```python
from build123d import *

# Parameters (mm, degrees)
SKETCH1_W                    = 139.7
SKETCH1_H                    = 457.2
SKETCH1_R                    = 50.8
SKETCH1_R_2                  = 5.08
BOSS_EXTRUDE1_DEPTH          = 9.652
SKETCH4_W                    = 10.452383168
SKETCH4_H                    = 6.858
SKETCH4_W_2                  = 8.864883168
SKETCH4_H_2                  = 6.35
CUT_EXTRUDE1_DEPTH           = 10.652
CHAMFER1_SIZE                = 15.24
CHAMFER1_SIZE2               = 30.48
CHAMFER2_SIZE                = 30.48
CHAMFER2_SIZE2               = 15.24
FILLET2_R                    = 15.24
SKETCH5_W                    = 76.2
SKETCH5_H                    = 9.652
BOSS_EXTRUDE2_DEPTH          = 4.318
F_3_0_3_DIAMETER_HOLE1_D     = 3
F_3_0_3_DIAMETER_HOLE1_DEPTH = 9.652


with BuildPart() as part:
    # Sketch1 → Boss-Extrude1 (new body)
    with BuildSketch(Plane(origin=(0, 0, 0), x_dir=(1, 0, 0), z_dir=(0, 1, 0))):
        with Locations((69.85, 228.6)):
            Rectangle(SKETCH1_W, SKETCH1_H)
        with Locations((63.5, 125.73)):
            Circle(SKETCH1_R, mode=Mode.SUBTRACT)
        with Locations((38.1, 38.1)):
            Circle(SKETCH1_R_2, mode=Mode.SUBTRACT)
        with Locations((38.1, 419.1)):
            Circle(SKETCH1_R_2, mode=Mode.SUBTRACT)
        with Locations((63.5, 331.47)):
            Circle(SKETCH1_R, mode=Mode.SUBTRACT)
        with Locations((38.1, 228.6)):
            Circle(SKETCH1_R_2, mode=Mode.SUBTRACT)
    extrude(amount=BOSS_EXTRUDE1_DEPTH)

    # Sketch4 → Cut-Extrude1 (cut, through all)
    with BuildSketch(Plane(origin=(0, 9.652, 0), x_dir=(1, 0, 0), z_dir=(0, 1, 0))):
        with Locations((5.226191584, 3.429)):
            Rectangle(SKETCH4_W, SKETCH4_H)
        with Locations((4.432441584, 454.025)):
            Rectangle(SKETCH4_W_2, SKETCH4_H_2)
    extrude(amount=-CUT_EXTRUDE1_DEPTH, mode=Mode.SUBTRACT)

    # Chamfer1
    chamfer1_edges = [part.edges().sort_by_distance(p)[0] for p in [
        (139.7, 4.826, -457.2),
    ]]
    chamfer1_side = [part.faces().sort_by_distance(p)[0] for p in [
        (139.7, 4.826, -228.6),
    ]]
    chamfer(chamfer1_edges, length=CHAMFER1_SIZE, length2=CHAMFER1_SIZE2, reference=chamfer1_side[0])

    # Chamfer2
    chamfer2_edges = [part.edges().sort_by_distance(p)[0] for p in [
        (139.7, 4.826, 0),
    ]]
    chamfer2_side = [part.faces().sort_by_distance(p)[0] for p in [
        (75.076191584, 4.826, 0),
    ]]
    chamfer(chamfer2_edges, length=CHAMFER2_SIZE, length2=CHAMFER2_SIZE2, reference=chamfer2_side[0])

    # Fillet2
    fillet2_edges = [part.edges().sort_by_distance(p)[0] for p in [
        (109.22, 4.826, -457.2),
        (109.22, 4.826, 0),
    ]]
    fillet(fillet2_edges, radius=FILLET2_R)

    # Sketch5 → Boss-Extrude2 (add)
    with BuildSketch(Plane(origin=(139.7, 0, 0), x_dir=(0, 0, -1), z_dir=(1, 0, 0))):
        with Locations((69.85, 4.826)):
            Rectangle(SKETCH5_W, SKETCH5_H)
        with Locations((228.6, 4.826)):
            Rectangle(SKETCH5_W, SKETCH5_H)
        with Locations((387.35, 4.826)):
            Rectangle(SKETCH5_W, SKETCH5_H)
    extrude(amount=BOSS_EXTRUDE2_DEPTH)

    # Ø3.0 (3) Diameter Hole1
    with Locations(Plane(origin=(0, 9.652, 0), x_dir=(1, 0, 0), z_dir=(0, 1, 0))):
        with Locations((101.092, 87.884), (25.4, 87.884), (25.4, 163.576), (101.092, 163.576)):
            f_3_0_3_diameter_hole1 = Hole(F_3_0_3_DIAMETER_HOLE1_D / 2, depth=F_3_0_3_DIAMETER_HOLE1_DEPTH)

    # Mirror1: Ø3.0 (3) Diameter Hole1 across plane
    add(f_3_0_3_diameter_hole1.mirror(Plane.XY.offset(-228.6)), mode=Mode.SUBTRACT)


solid = part.part
```
The listing builds one solid part. Answer for the finished solid, in the listing's coordinates (mm). A direction names the side the tool comes from. Coordinates: 2 decimals unless noted, no trailing zeros. Loops run counter-clockwise (first coordinate to the right, second up) from the corner with the lowest first, then second, coordinate; pieces in that order, holes last. Notation, with made-up numbers: (-36, -31) - (9, -31) arc R9 ccw to (9, -24) - close; hole circle Ø9 at (52, -31). An arc over 180 degrees is marked (long way). Use a Markdown table: item, result. Add a question column.
1) The part is cut by section A-A, the plane z = -228.6. Give the vertices of the cut face in (x, y).
2) Given pin 1 (2.5 mm diameter, centred on x = 101.092, z = -369.316, fed in from +Y); pin 2 (5 mm diameter, centred on y = 5, z = -23.5, fed in from +X); pin 3 (1.3 mm diameter, centred on x = 141, y = 3, fed in from -Z); pin 4 (5.5 mm diameter, centred on y = 6, z = -3.5, fed in from -X), each flat-ended and moving along its own axis, determine where each tip first touches the part or whether it passes through.
3) The part is cut by section D-D, the plane x = 38.1. Give the vertices of the cut face in (y, z).
4) The part is cut by section C-C, the plane z = -331.47. Give the vertices of the cut face in (x, y), and give its area (3 significant figures).
5) The part is cut by section B-B, the plane x = 63.5. Give the vertices of the cut face in (y, z), and give its area (3 significant figures).
6) The mould has two halves that part along Z. Classify faces 1 (the flat face through (126.26, 4.76, -8.52)), 2 (the flat face through (139.7, 5, -434)), 3 (the cylindrical face through (26, 5, -160)): released by +Z, released by -Z, zero draft, split by the parting line, or undercut.
7) For faces 4 (the flat face through (4, 5, -450.85)), 5 (the flat face through (139.7, 5, -307)), 6 (the flat face through (5, 5, -6.858)), 7 (the flat face through (139.7, 5, -23)), determine the directions among +Z, -Z, +X, -X, +Y, -Y from which every point of the face is accessible in a straight line to the end or side of a thin tool.
8) Find the intervals of material crossed by line 1 (Z direction, x = 63.5, y = 2); line 2 (X direction, y = 7.5, z = -331.47); line 3 (X direction, y = 3, z = -38.1), in increasing order.
Here are the results:
| question | item | result |
|---|---|---|
| 1 | outline | (0, 0) - (33.02, 0) - (33.02, 9.65) - (0, 9.65) - close; (43.18, 0) - (144.02, 0) - (144.02, 9.65) - (43.18, 9.65) - close |
| 2 | pin 1 | passes through |
| 2 | pin 2 | stops at x = 139.7 |
| 2 | pin 3 | stops at z = -425.45 |
| 2 | pin 4 | stops at x = 10.45 |
| 3 | outline | (0, -457.2) - (9.65, -457.2) - (9.65, -424.18) - (0, -424.18) - close; (0, -414.02) - (9.65, -414.02) - (9.65, -375.46) - (0, -375.46) - close; (0, -287.48) - (9.65, -287.48) - (9.65, -233.68) - (0, -233.68) - close; (0, -223.52) - (9.65, -223.52) - (9.65, -169.72) - (0, -169.72) - close; (0, -81.74) - (9.65, -81.74) - (9.65, -43.18) - (0, -43.18) - close; (0, -33.02) - (9.65, -33.02) - (9.65, 0) - (0, 0) - close |
| 4 | outline | (0, 0) - (12.7, 0) - (12.7, 9.65) - (0, 9.65) - close; (114.3, 0) - (139.7, 0) - (139.7, 9.65) - (114.3, 9.65) - close |
| 4 | area | 368 mm^2 |
| 5 | outline | (0, -457.2) - (9.65, -457.2) - (9.65, -382.27) - (0, -382.27) - close; (0, -280.67) - (9.65, -280.67) - (9.65, -176.53) - (0, -176.53) - close; (0, -74.93) - (9.65, -74.93) - (9.65, 0) - (0, 0) - close |
| 5 | area | 2,450 mm^2 |
| 6 | face 1 | released by +Z |
| 6 | face 2 | zero draft |
| 6 | face 3 | undercut |
| 7 | face 4 | -Z, -X, +Y, -Y |
| 7 | face 5 | +X, +Y, -Y |
| 7 | face 6 | +Z, -X, +Y, -Y |
| 7 | face 7 | +Z, +X, +Y, -Y |
| 8 | line 1 | z = -457.2 to -382.27, -280.67 to -176.53, -74.93 to 0 |
| 8 | line 2 | x = 0 to 12.7, 114.3 to 139.7 |
| 8 | line 3 | x = 0 to 33.02, 43.18 to 144.02 |
